Could you check a few things on this model? Use its own coordinates, in mm. Give positions to 0.01 mm unless a question says otherwise; leave off trailing zeros. Order: outer loops, then holes, each group sorted by start corner. A loop starts at its lowest first (then second) coordinate and runs counter-clockwise, first axis right, second up. Notation, with made-up numbers: M 49.25,-34.5 L 81.25,-34.5 A20 ccw 81.25,-29.5 Z; hole C 49.5,68 d8. An arc over 180 degrees is marked long. Use a Markdown table: item, result. Add a question column.
Item 1: If I drill on L1, parallel to Y at x = -0.4, z = 0.1; L2, parallel to Z at x = 0, y = 5.25; L3, parallel to X at y = 0.75, z = 0.2, over which ranges is the centre line in solid material (lowest first)? Write a range as from..to.
Item 2: Suppose I cut it at C-C on y = -0.25. Write out the boundary of the cut face in (x, z).
Item 3: Suppose I cut it at B-B on x = 0. Write out the boundary of the cut face in (y, z), plus the area to 3 significant figures.
Item 4: Suppose I cut it at A-A on z = 0. Write out the boundary of the cut face in (x, y), plus the area to 3 significant figures.
from build123d import *

# Parameters (mm, degrees)
SKETCH2_R           = 0.3
BASE_EXTRUDE_DEPTH  = 6.5
SKETCH3_R           = 0.5
BOSS_EXTRUDE1_DEPTH = 0.5
SKETCH4_R           = 0.3
BOSS_EXTRUDE2_DEPTH = 3


with BuildPart() as part:
    # Sketch2 → Base-Extrude (new body)
    with BuildSketch(Plane(origin=(0, 0, 0), x_dir=(1, 0, 0), z_dir=(0, 1, 0))):
        Circle(SKETCH2_R)
    extrude(amount=BASE_EXTRUDE_DEPTH)

    # Sketch3 → Boss-Extrude1 (add)
    with BuildSketch(Plane.XZ):
        Circle(SKETCH3_R)
    extrude(amount=-BOSS_EXTRUDE1_DEPTH)

    # Sketch4 → Boss-Extrude2 (add)
    with BuildSketch(Plane.XZ):
        Circle(SKETCH4_R)
    extrude(amount=BOSS_EXTRUDE2_DEPTH)


solid = part.part
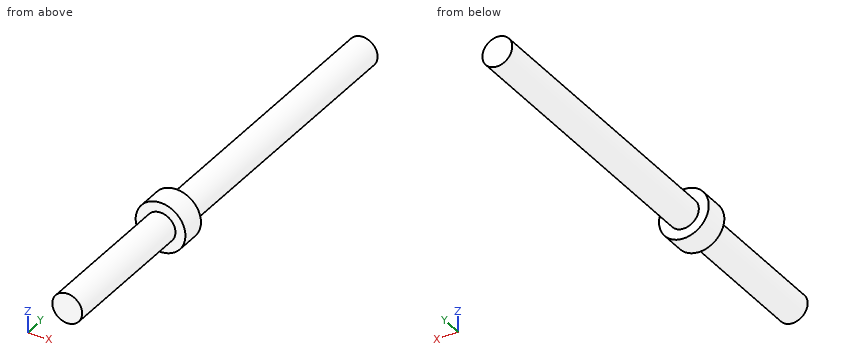
Findings below:
| question | item | result |
|---|---|---|
| 1 | L1 | y = 0..0.5 |
| 1 | L2 | z = -0.3..0.3 |
| 1 | L3 | x = -0.22..0.22 |
| 2 | outline | C 0,0 d0.6 |
| 3 | outline | M -3,-0.3 L 0,-0.3 L 0,-0.5 L 0.5,-0.5 L 0.5,-0.3 L 6.5,-0.3 L 6.5,0.3 L 0.5,0.3 L 0.5,0.5 L 0,0.5 L 0,0.3 L -3,0.3 Z |
| 3 | area | 5.90 mm^2 |
| 4 | outline | M -0.5,0 L -0.3,0 L -0.3,-3 L 0.3,-3 L 0.3,0 L 0.5,0 L 0.5,0.5 L 0.3,0.5 L 0.3,6.5 L -0.3,6.5 L -0.3,0.5 L -0.5,0.5 Z |
| 4 | area | 5.90 mm^2 |
